Autodesk Inventor part; units mm, degrees
ref_plane "YZ Plane" through (0, 0, 0) normal (1, 0, 0) x (0, 1, 0)
ref_plane "XZ Plane" through (0, 0, 0) normal (0, 1, 0) x (-1, 0, 0)
ref_plane "XY Plane" through (0, 0, 0) normal (0, 0, 1) x (1, 0, 0)
sketch "Skizze1" plane through (0, 0, 0) normal (1, 0, 0) x (0, 1, 0)
  line L0 (0, 0) -> (30, 0)
  line L1 (30, 0) -> (30, -39)
  line L2 (30, -39) -> (0, -39)
  line L3 (0, -39) -> (0, 0)
  dimension "d0" = 30
  dimension "d1" = 39
extrude "Extrusion1" add sketch "Skizze1" along normal blind 2
sketch "Skizze2" plane through (2, 0, 0) normal (1, 0, 0) x (0, 0, -1)
  line L0 (2.2, 27.8) -> (36.8, 27.8)
  line L1 (36.8, 27.8) -> (36.8, 2.2)
  line L2 (36.8, 2.2) -> (2.2, 2.2)
  line L3 (2.2, 2.2) -> (2.2, 27.8)
  line L4 (0, 30) -> (0, 0)
  line L5 (39, 30) -> (0, 30)
  dimension "d4" = 25.6
  dimension "d5" = 34.6
  dimension "d6" = 2.2
  dimension "d7" = 2.2
extrude "Extrusion2" add sketch "Skizze2" along normal blind 2
chamfer "Fase1" distance 0.5 angle 45 4 edges at (4, 27.8, -19.5) (4, 15, -2.2) (4, 2.2, -19.5) (4, 15, -36.8)
sketch "Skizze3" plane through (0, 0, 0) normal (-1, 0, 0) x (0, 0, 1)
  line L0 (0, 0) -> (-39, 0)
  line L1 (0, 0) -> (-9, 0)
  line L2 (-9, 0) -> (-9, -10)
  line L3 (-9, -10) -> (0, -10)
  line L4 (0, -10) -> (0, 0)
  line L5 (-39, 0) -> (-39, 30)
  line L6 (-39, 30) -> (-30, 30)
  line L7 (-30, 30) -> (-30, 40)
  line L8 (-30, 40) -> (-39, 40)
  line L9 (-39, 40) -> (-39, 30)
  circle A0 centre (-5, -5) radius 1.65
  circle A1 centre (-34, 35) radius 1.65
  dimension "d13" = 10
  dimension "d14" = 9
  dimension "d15" = 9
  dimension "d16" = 10
  dimension "d17" = 5
  dimension "d18" = 5
  dimension "d19" = 3.3
  dimension "d20" = 5
  dimension "d21" = 5
  dimension "d22" = 3.3
extrude "Extrusion3" add sketch "Skizze3" against normal blind 2
fillet "Rundung1" radius 2 8 edges at (1, -10, 0) (1, -10, -9) (1, 0, -39) (1, 40, -39) (1, 0, -9) (1, 40, -30) (1, 30, -30) (1, 30, 0)
properties part number "deckel_wemos"
Source: CAD feature listing. Evaluate the final solid. Frame: model axes, mm. A direction names the side the tool comes from. Give positions to 0.01 mm unless a question says otherwise; leave off trailing zeros. Loops run counter-clockwise (first coordinate to the right, second up) from the corner with the lowest first, then second, coordinate; pieces in that order, holes last. Notation, with made-up numbers: (-6.5, -10.75) -> (22.5, -10.75) arc R4 ccw to (22.5, -3.75) -> close; hole circle Ø10 at (39.25, 17). An arc over 180 degrees is marked (long way). Use a Markdown table: item, result. Add a question column.
(1) First-contact query: pin 1 Ø0.8 at (x, y) = (3, 10.5) entering from -Z; pin 2 Ø1 at (x, y) = (1, 35) entering from +Z; pin 3 Ø0.6 at (x, z) = (1.5, -11.5) entering from +Y. Flat tips, straight axial feed; report the tip coordinate or a pass-through.
(2) Section query C-C (y = -5). Output: boundary loops of the cut face in (x, z), then the cut area to 3 significant figures.
(3) Section query B-B (x = 1.2). Output: boundary loops of the cut face in (y, z), then the cut area to 3 significant figures.
(4) Section query D-D (y = 6). Output: boundary loops of the cut face in (x, z), then the cut area to 3 significant figures.
(5) Access query for faces 4 (the face through (3, 2.2, -20)), 5 (the face through (3, 15, -2.2)), 6 (the face through (1, 0, -24)). Directions: +Z, -Z, +X, -X, +Y, -Y. A direction counts if a zero-diameter tool reaches every point of the face in a straight line with its end or side. Return the directions, or none.
(6) Pull-direction query (Z, two-part tool) for faces 1 (the face through (0.986, 36.115, -35.216)), 2 (the face through (1.01, -9.4, -0.57)), 3 (the face through (1, 30, -15)); classes: +Z half, -Z half, draft (parallel to the pull), parting line (faces both ways), or undercut.
(7) Ray query, line 1 (Y direction, x = 1, z = -34); line 2 (Y direction, x = 0.5, z = -5); line 3 (X direction, y = 30, z = -30.5). Return the intervals inside material, ascending.
(8) Section query A-A (z = -5). Output: boundary loops of the cut face in (x, y), then the cut area to 3 significant figures.
Checked values:
| question | item | result |
|---|---|---|
| 1 | pin 1 | z = -36.8 |
| 1 | pin 2 | z = -30 |
| 1 | pin 3 | y = 30 |
| 2 | outline | (0, -9) -> (2, -9) -> (2, -6.65) -> (0, -6.65) -> close; (0, -3.35) -> (2, -3.35) -> (2, 0) -> (0, 0) -> close |
| 2 | area | 11.4 mm^2 |
| 3 | outline | (-10, -7) arc R2 ccw to (-8, -9) -> (-2, -9) arc R2 cw to (0, -11) -> (0, -37) arc R2 ccw to (2, -39) -> (38, -39) arc R2 ccw to (40, -37) -> (40, -32) arc R2 ccw to (38, -30) -> (32, -30) arc R2 cw to (30, -28) -> (30, -2) arc R2 ccw to (28, 0) -> (-8, 0) arc R2 ccw to (-10, -2) -> close; hole circle Ø3.3 at (-5, -5); hole circle Ø3.3 at (35, -34) |
| 3 | area | 1,330 mm^2 |
| 4 | outline | (0, -39) -> (2, -39) -> (2, -36.8) -> (3.5, -36.8) -> (4, -36.3) -> (4, -2.7) -> (3.5, -2.2) -> (2, -2.2) -> (2, 0) -> (0, 0) -> close |
| 4 | area | 147 mm^2 |
| 5 | face 4 | +Z, -Z, +X, -Y |
| 5 | face 5 | +Z, +X, +Y, -Y |
| 5 | face 6 | -Z, +X, -X, -Y |
| 6 | face 1 | undercut |
| 6 | face 2 | +Z half |
| 6 | face 3 | draft |
| 7 | line 1 | 0 to 33.35, 36.65 to 40 |
| 7 | line 2 | -10 to -6.65, -3.35 to 30 |
| 7 | line 3 | 0 to 2 |
| 8 | outline | (0, -10) -> (2, -10) -> (2, -6.65) -> (0, -6.65) -> close; (0, -3.35) -> (2, -3.35) -> (2, 2.2) -> (3.5, 2.2) -> (4, 2.7) -> (4, 27.3) -> (3.5, 27.8) -> (2, 27.8) -> (2, 30) -> (0, 30) -> close |
| 8 | area | 124 mm^2 |
